from build123d import *

# Parameters (mm, degrees)
SKETCH1_W                                      = 60.6552
SKETCH1_H                                      = 128.4986
BOSS_EXTRUDE1_DEPTH                            = 2.54
CSK_FOR_M3_FLAT_HEAD_MACHINE_SCREW1_AT_2_COUNT = 2
CSK_FOR_M3_FLAT_HEAD_MACHINE_SCREW1_AT_2_PITCH = 75.0062
M2_5_CLEARANCE_SLOT1_DEPTH                     = 2.54
F_1_4_CLEARANCE_HOLE1_D                        = 7.14248
F_1_4_CLEARANCE_HOLE2_D                        = 6.5278
F_3_8_CLEARANCE_HOLE2_D                        = 10.0838
F_10_CLEARANCE_HOLE1_D                         = 5.6134
CSK_FOR_M2_5_FLAT_HEAD_MACHINE_SCREW1_AT_COUNT = 2
CSK_FOR_M2_5_FLAT_HEAD_MACHINE_SCREW1_AT_PITCH = 35.56
F_11_64_0_17188_DIAMETER_HOLE1_D               = 4.365752


# Read off the part's stored shape, not the designer's step: M2.5 Clearance Slot1
with BuildPart() as part:
    # Sketch1 → Boss-Extrude1 (new body)
    with BuildSketch(Plane(origin=(0, 0, 0), x_dir=(1, 0, 0), z_dir=(0, 1, 0))):
        Rectangle(SKETCH1_W, SKETCH1_H)
    extrude(amount=BOSS_EXTRUDE1_DEPTH)

    # Sketch5 → CSK for M3 Flat Head Machine Screw1 (revolve, cut)
    with BuildSketch(Plane(origin=(25.4, 0, -37.5031), x_dir=(0, 0, -1), z_dir=(1, 0, 0))):
        Polygon((0, 0), (0, 2.54), (1.8, 2.54), (1.8, 1.35), (3.15, 0), align=None)
    csk_for_m3_flat_head_machine_screw1 = revolve(axis=Axis((25.4, -6.35, -37.5031), (0, 1, 0)), mode=Mode.SUBTRACT)

    # CSK for M3 Flat Head Machine Screw1 at 2: CSK for M3 Flat Head Machine Screw1 ×2
    with Locations(*[(0, 0, i * CSK_FOR_M3_FLAT_HEAD_MACHINE_SCREW1_AT_2_PITCH) for i in range(1, CSK_FOR_M3_FLAT_HEAD_MACHINE_SCREW1_AT_2_COUNT)]):
        add(csk_for_m3_flat_head_machine_screw1, mode=Mode.SUBTRACT)

    # M2.5 Clearance Slot1 outline → M2.5 Clearance Slot1 (cut)
    with BuildSketch(Plane(origin=(0, 0, 0), x_dir=(1, 0, 0), z_dir=(0, 1, 0))):
        with BuildLine():
            ThreePointArc((23.36, -62.7021), (24.81, -61.2521), (23.36, -59.8021))
            Line((23.36, -59.8021), (22.36, -59.8021))
            ThreePointArc((22.36, -59.8021), (20.91, -61.2521), (22.36, -62.7021))
            Line((22.36, -62.7021), (23.36, -62.7021))
        make_face()
        with BuildLine():
            ThreePointArc((23.36, 59.8021), (24.81, 61.2521), (23.36, 62.7021))
            Line((23.36, 62.7021), (22.36, 62.7021))
            ThreePointArc((22.36, 62.7021), (20.91, 61.2521), (22.36, 59.8021))
            Line((22.36, 59.8021), (23.36, 59.8021))
        make_face()
    m2_5_clearance_slot1 = extrude(amount=M2_5_CLEARANCE_SLOT1_DEPTH, mode=Mode.SUBTRACT)

    # Mirror1: CSK for M3 Flat Head Machine Screw1, M2.5 Clearance Slot1 across plane
    add(csk_for_m3_flat_head_machine_screw1.mirror(Plane(origin=(0, 0, 0), x_dir=(0, 0, 1), z_dir=(1, 0, 0))), mode=Mode.SUBTRACT)
    add(m2_5_clearance_slot1.mirror(Plane(origin=(0, 0, 0), x_dir=(0, 0, 1), z_dir=(1, 0, 0))), mode=Mode.SUBTRACT)

    # Mirror1 copy 1 sketch → Mirror1 copy 1 (revolve, cut)
    with BuildSketch(Plane(origin=(-25.4, 0, 37.5031), x_dir=(0, 0, -1), z_dir=(-1, 0, 0))):
        Polygon((0, 0), (0, -2.54), (1.8, -2.54), (1.8, -1.35), (3.15, 0), align=None)
    revolve(axis=Axis((-25.4, -6.35, 37.5031), (0, -1, 0)), mode=Mode.SUBTRACT)

    # 1/4 Clearance Hole1 (through all)
    with Locations(Plane(origin=(0, 0, 0), x_dir=(-1, 0, 0), z_dir=(0, -1, 0))):
        with Locations((16.3576, 35.0012), (16.3576, 21.301199968), (16.3576, -32.798800036)):
            Hole(F_1_4_CLEARANCE_HOLE1_D / 2)

    # 1/4 Clearance Hole2 (through all)
    with Locations(Plane(origin=(0, 0, 0), x_dir=(-1, 0, 0), z_dir=(0, -1, 0))):
        with Locations((-12.2174, 35.0012), (2.0701, 35.0012), (2.0701, 21.301199968), (-12.2174, 21.301199968), (-12.2174, -17.08879996), (2.0701, -32.798800036)):
            Hole(F_1_4_CLEARANCE_HOLE2_D / 2)

    # 3/8 Clearance Hole2 (through all)
    with Locations(Plane(origin=(0, 0, 0), x_dir=(-1, 0, 0), z_dir=(0, -1, 0))):
        with Locations((9.7536, -17.08879996), (-5.07365, 2.731200024)):
            Hole(F_3_8_CLEARANCE_HOLE2_D / 2)

    # #10 Clearance Hole1 (through all)
    with Locations(Plane(origin=(0, 0, 0), x_dir=(-1, 0, 0), z_dir=(0, -1, 0))):
        with Locations((-12.2174, -32.798800036)):
            Hole(F_10_CLEARANCE_HOLE1_D / 2)

    # Sketch73 → CSK for M2.5 Flat Head Machine Screw1 (revolve, cut)
    with BuildSketch(Plane(origin=(-17.78, 2.54, 49.2633), x_dir=(0, 0, 1), z_dir=(1, 0, 0))):
        Polygon((0, 0), (0, 2.54), (1.45, 2.54), (1.45, 1.3), (2.75, 0), align=None)
    csk_for_m2_5_flat_head_machine_screw1 = revolve(axis=Axis((-17.78, 8.89, 49.2633), (0, -1, 0)), mode=Mode.SUBTRACT)

    # CSK for M2.5 Flat Head Machine Screw1 at: CSK for M2.5 Flat Head Machine Screw1 ×2
    with Locations(*[(i * CSK_FOR_M2_5_FLAT_HEAD_MACHINE_SCREW1_AT_PITCH, 0, 0) for i in range(1, CSK_FOR_M2_5_FLAT_HEAD_MACHINE_SCREW1_AT_COUNT)]):
        add(csk_for_m2_5_flat_head_machine_screw1, mode=Mode.SUBTRACT)

    # 11/64 (0.17188) Diameter Hole1 (through all)
    with Locations(Plane(origin=(0, 0, 0), x_dir=(-1, 0, 0), z_dir=(0, -1, 0))):
        with Locations((11.938, 9.731199994), (11.938, 2.731200024), (11.938, -4.268799946)):
            Hole(F_11_64_0_17188_DIAMETER_HOLE1_D / 2)


solid = part.part
Can you work these out from the model? Positions are in its coordinate system, mm. A direction names the side the tool comes from. Give positions to 0.01 mm unless a question says otherwise; leave off trailing zeros. Order: outer loops, then holes, each group sorted by start corner. A loop starts at its lowest first (then second) coordinate and runs counter-clockwise, first axis right, second up. Notation, with made-up numbers: M 55.5,72 L 62.5,72 A21 cw 62.5,91 Z; hole C -32,71.25 d10. An arc over 180 degrees is marked long. Use a Markdown table: item, result. Add a question column.
Item 1: Suppose I cut it at A-A (x = 17.78). List the corners of the cut face in (y, z) for me.
Item 2: For faces 1 (the cylindrical face through (-24.81, 1.25, 61.28)), 2 (the flat face through (0, 2.54, -1)), which set-ups out of +Z, -Z, +X, -X, +Y, -Y let a thin tool reach every point of the face, with its end or its side?
Item 3: Will these pins go through, and if not, where does the flat tip stop? pin 1 (2.5 mm diameter, centred on x = -17.78, z = 49.26, fed in from +Y); pin 2 (13 mm diameter, centred on x = 5.07, z = -2.73, fed in from +Y).
Item 4: If I drill on L1, parallel to Z at x = -17.78, y = 0.8; L2, parallel to X at y = 0.1, z = -21; L3, parallel to Z at x = 24.5, y = 0.4, over which ranges is the centre line in solid material (lowest first)? Write a range as [from, to].
Item 5: We'd pull the mould along Z, two halves only. Please class faces 3 (the cylindrical face through (-19.925, 1.288, 32.642)), 4 (the cylindrical face through (-0.564, 1.288, -18.406)), 5 (the flat face through (-30.328, 1, 1)), 6 (the flat face through (0, 1, -64.249)): +Z half, -Z half, draft (parallel to the pull), parting line (faces both ways), or undercut.
Item 6: Suppose I cut it at C-C (y = 2). Count the separate pieces of the cut face and the enclosed holes in it, then the cut area to 3 significant figures.
Item 7: Suppose I cut it at B-B (x = -7.5). List the corners of the cut face in (y, z) for me.
Answer sheet:
| question | item | result |
|---|---|---|
| 1 | outline | M 0,-64.25 L 2.54,-64.25 L 2.54,46.51 L 1.24,47.81 L 0,47.81 Z; M 0,50.71 L 1.24,50.71 L 2.54,52.01 L 2.54,64.25 L 0,64.25 Z |
| 2 | face 1 | +Y, -Y |
| 2 | face 2 | +Z, -Z, +X, -X, +Y |
| 3 | pin 1 | passes through |
| 3 | pin 2 | stops at y = 2.54 |
| 4 | L1 | z = [-64.25, -38.28], [-31.73, -24.58], [-18.03, 29.52], [36.07, 47.81], [50.71, 64.25] |
| 4 | L2 | x = [-30.33, -19.92], [-12.8, -5.32], [1.18, 8.97], [15.47, 30.33] |
| 4 | L3 | z = [-64.25, -62.15], [-60.36, -40.1], [-34.9, 34.9], [40.1, 60.36], [62.15, 64.25] |
| 5 | face 3 | undercut |
| 5 | face 4 | undercut |
| 5 | face 5 | draft |
| 5 | face 6 | -Z half |
| 6 | separate pieces | 1 |
| 6 | enclosed holes | 25 |
| 6 | area | 7,130 mm² |
| 7 | outline | M 0,-64.25 L 2.54,-64.25 L 2.54,12.58 L 0,12.58 Z; M 0,21.6 L 2.54,21.6 L 2.54,64.25 L 0,64.25 Z |
